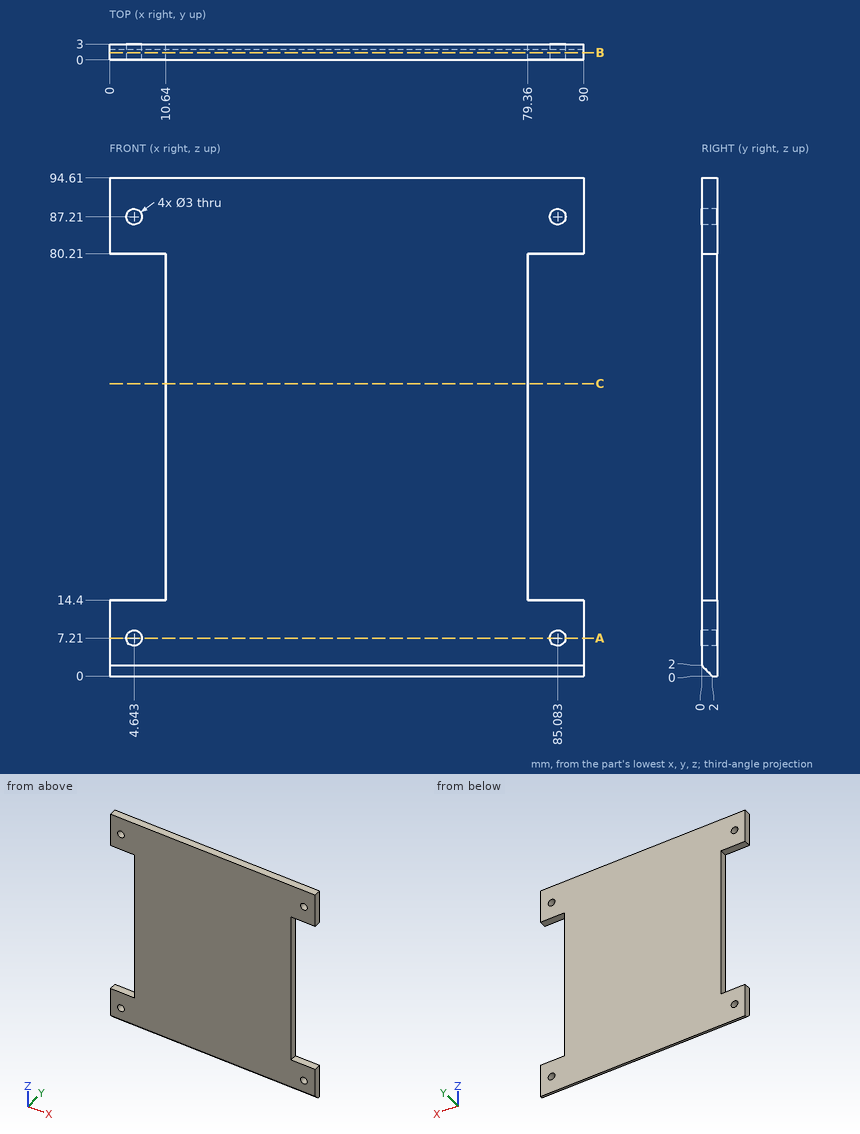
Source: three-view drawing plus pictorial views. Frame: mm from the lowest corner of the part. Give positions to 0.01 mm unless a question says otherwise; leave off trailing zeros. Order: outer loops, then holes, each group sorted by start corner. A loop starts at its lowest first (then second) coordinate and runs counter-clockwise, first axis right, second up. Notation, with made-up numbers: (38.25, -20.75) - (77.25, -20.75) arc R8 ccw to (77.25, -7.75) - close; hole circle Ø4 at (65.5, 0). An arc over 180 degrees is marked (long way). Answer as a JSON object with one key per item and string values. Group by question number.
Q1. Cut plane A-A, the plane z = 7.21. Output: boundary loops of the cut face in (x, y), then the cut area to 3 significant figures.
Q2. Cut plane C-C, the plane z = 55.5. Output: boundary loops of the cut face in (x, y).
Q3. First-contact query: pin 1 Ø1 at (y, z) = (1.5, 27.5) entering from +X; pin 2 Ø1 at (y, z) = (1.5, 25) entering from -X. Flat tips, straight axial feed; report the tip coordinate or a pass-through.
Q4. Cut plane B-B, the plane y = 1.35. Output: boundary loops of the cut face in (x, z), then the cut area to 3 significant figures.
Q5. Line query: probe 1 along Z at (x, y) = (6, 1); probe 2 along X at (y, z) = (1.05, 78.5); probe 3 along Z at (x, y) = (79.5, 2.3). Output: solid intervals per line, ascending.
Results:
{
 "1": {"outline": "(0, 0) - (3.14, 0) - (3.14, 3) - (0, 3) - close; (6.14, 0) - (83.58, 0) - (83.58, 3) - (6.14, 3) - close; (86.58, 0) - (90, 0) - (90, 3) - (86.58, 3) - close", "area": "252 mm^2"},
 "2": {"outline": "(10.64, 0) - (79.36, 0) - (79.36, 3) - (10.64, 3) - close"},
 "3": {"pin 1": "x = 79.36", "pin 2": "x = 10.64"},
 "4": {"outline": "(0, 0.65) - (90, 0.65) - (90, 14.4) - (79.36, 14.4) - (79.36, 80.21) - (90, 80.21) - (90, 94.61) - (0, 94.61) - (0, 80.21) - (10.64, 80.21) - (10.64, 14.4) - (0, 14.4) - close; hole circle Ø3 at (4.64, 7.21); hole circle Ø3 at (4.64, 87.21); hole circle Ø3 at (85.08, 7.21); hole circle Ø3 at (85.08, 87.21)", "area": "7,030 mm^2"},
 "5": {"probe 1": "1 to 6.57, 7.85 to 14.4, 80.21 to 86.57, 87.85 to 94.61", "probe 2": "10.64 to 79.36", "probe 3": "0 to 14.4, 80.21 to 94.61"}
}
